```python
from build123d import *

# Parameters (mm, degrees)
PAD001_DEPTH    = 10
SKETCH002_W     = 10
SKETCH002_H     = 30
PAD002_DEPTH    = 8
SKETCH003_R     = 4
POCKET_DEPTH    = 10
SKETCH004_R     = 2
POCKET001_DEPTH = 20
SKETCH005_R     = 2
POCKET002_DEPTH = 20


with BuildPart() as part:
    # Sketch001 → Pad001 (new body)
    with BuildSketch(Plane(origin=(0, 0, 0), x_dir=(1, 0, 0), z_dir=(0, 0, -1))):
        Polygon((-300, 190), (-280, 190), (-280, 160), (-220, 160), (-220, 120), (-300, 120), align=None)
    extrude(amount=PAD001_DEPTH)

    # Sketch002 → Pad002 (new body)
    with BuildSketch(Plane.XY):
        with Locations((-285, -175)):
            Rectangle(SKETCH002_W, SKETCH002_H)
    extrude(amount=PAD002_DEPTH)

    # Sketch003 → Pocket (cut)
    with BuildSketch(Plane.YZ.offset(-280)):
        with Locations((-175, 10)):
            Circle(SKETCH003_R)
    extrude(amount=-POCKET_DEPTH, mode=Mode.SUBTRACT)

    # Sketch004 → Pocket001 (cut)
    with BuildSketch(Plane.XY.offset(8)):
        with Locations((-285, -185)):
            Circle(SKETCH004_R)
    extrude(amount=-POCKET001_DEPTH, mode=Mode.SUBTRACT)

    # Sketch005 → Pocket002 (cut)
    with BuildSketch(Plane.XY.offset(8)):
        with Locations((-285, -165)):
            Circle(SKETCH005_R)
    extrude(amount=-POCKET002_DEPTH, mode=Mode.SUBTRACT)


solid = part.part
```
Input: part model. Units: mm. Frame: model coordinates. A direction names the side the tool comes from. Give positions to 0.01 mm unless a question says otherwise; leave off trailing zeros. Order: outer loops, then holes, each group sorted by start corner. A loop starts at its lowest first (then second) coordinate and runs counter-clockwise, first axis right, second up. Notation, with made-up numbers: (49, 53) - (63, 53) arc R24 ccw to (63, 76) - close; hole circle Ø2 at (23.5, 21.25). An arc over 180 degrees is marked (long way). One line per item, written item: value.
1. Cut plane D-D, the plane x = -240.5. Output: boundary loops of the cut face in (y, z).
Determined:
outline: (-160, -10) - (-120, -10) - (-120, 0) - (-160, 0) - close
2. Pin query (flat end, axial travel): pin 1 Ø4.5 at (x, y) = (-285, -185) entering from +Z; pin 2 Ø5 at (x, z) = (-243, -3.5) entering from -Y; pin 3 Ø3 at (x, y) = (-230.5, -135.5) entering from +Z; pin 4 Ø12 at (x, y) = (-262, -171) entering from +Z. Return the tip coordinate at first contact, or that it passes through.
Determined:
pin 1: z = 8
pin 2: y = -160
pin 3: z = 0
pin 4: through
3. Cut plane C-C, the plane y = -165. Output: boundary loops of the cut face in (x, z), and give its area (3 significant figures).
Determined:
outline: (-300, -10) - (-287, -10) - (-287, 8) - (-290, 8) - (-290, 0) - (-300, 0) - close; (-283, -10) - (-280, -10) - (-280, 8) - (-283, 8) - close
area: 208 mm2
4. Line query: probe 1 along Y at (x, z) = (-285, 1.5); probe 2 along Y at (x, z) = (-285, -2); probe 3 along X at (y, z) = (-165, -0.5). Output: solid intervals per line, ascending.
Determined:
probe 1: -190 to -187, -183 to -167, -163 to -160
probe 2: -190 to -187, -183 to -167, -163 to -120
probe 3: -300 to -287, -283 to -280
5. Cut plane B-B, the plane z = -1.75. Output: boundary loops of the cut face in (x, y), and give its area (3 significant figures).
Determined:
outline: (-300, -190) - (-280, -190) - (-280, -160) - (-220, -160) - (-220, -120) - (-300, -120) - close; hole circle Ø4 at (-285, -185); hole circle Ø4 at (-285, -165)
area: 3,770 mm2
6. Reachability of faces 4 (the face through (-285, -160, 4)), 5 (the face through (-259, -148, -10)), 6 (the face through (-250, -160, -5)) from +Z, -Z, +X, -X, +Y, -Y: full face, straight path, thin tool, end or side. Return the list, or none.
Determined:
face 4: +Z, +X, -X, +Y
face 5: -Z, +X, -X, +Y, -Y
face 6: +Z, -Z, +X, -Y
7. Draft query along X for faces 1 (the face through (-290, -175, 4)), 2 (the face through (-220, -140, -5)), 3 (the face through (-286.6, -166.2, -0.9)). Return one class per face: released by +X, released by -X, zero draft, split by the parting line, or undercut.
Determined:
face 1: released by -X
face 2: released by +X
face 3: undercut
8. Cut plane A-A, the plane x = -285. Output: boundary loops of the cut face in (y, z), and give its area (3 significant figures).
Determined:
outline: (-190, -10) - (-187, -10) - (-187, 8) - (-190, 8) - close; (-183, -10) - (-167, -10) - (-167, 8) - (-171.54, 8) arc R4 cw to (-178.46, 8) - (-183, 8) - close; (-163, -10) - (-120, -10) - (-120, 0) - (-160, 0) - (-160, 8) - (-163, 8) - close
area: 786 mm2
